Can you work these out from the model? Positions are in its coordinate system, mm. Face numbers are marked on the shaded views. A direction names the side the tool comes from. Round coordinates to 2 decimals unless told otherwise and drop trailing zeros.
Q1. For the marked faces 1 and 2, which set-ups out of +Z, -Z, +X, -X, +Y, -Y let a thin tool reach every point of the face, with its end or its side?
Q2. Will these pins go through, and if not, where does the flat tip stop? P1, Ø1.5, axis at y = 25, z = 1, coming from the -X side; P2, Ø3, axis at x = 15.5, z = 6, coming from the +Y side; P3, Ø2, axis at x = -1, z = 4.5, coming from the -Y side.
Q3. We'd pull the mould along X, two halves only. Please class the marked faces 3 and 4: pulls with the +X half, pulls with the -X half, needs draft (parallel to the pull), parting line crosses it, or undercut.
Q4. If we section it at A-A (x = 7.5): Count the separate pieces of the cut face and the enclosed holes in it, plus the area to 3 significant figures.
Q5. If I drill on line 1 (X direction, y = -0.5, z = 4.5); line 2 (Y direction, x = 7.5, z = 4); line 3 (Z direction, x = 22, y = 19.5), over which ranges is the centre line in solid material (lowest first)?
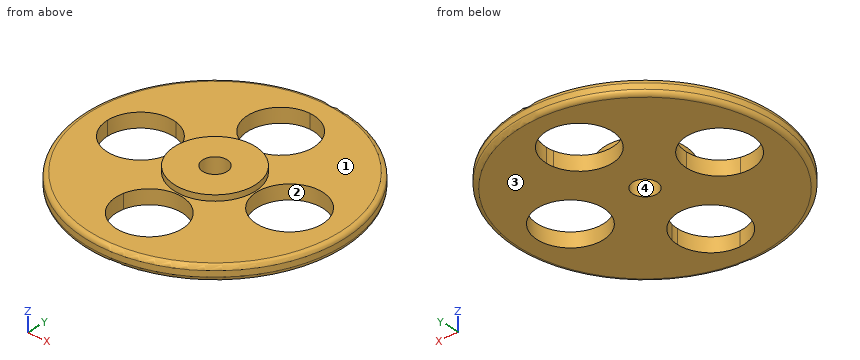
from build123d import *

# Parameters (mm, degrees)
F0_R     = 45
F0_R_2   = 14
F1_DEPTH = 5
F0_R_3   = 4.25
F2_DEPTH = 7
F3_R     = 1.5


with BuildPart() as f1:
    # F0 (on Top) → F1 (new body)
    with BuildSketch(Plane.XY):
        Circle(F0_R)
        with BuildLine():
            ThreePointArc((0, 37.5), (26.5165042945, 26.5165042945), (37.5, 0))
            ThreePointArc((37.5, 0), (26.5165043235, -26.5165042654), (8.22e-08, -37.5))
            ThreePointArc((8.22e-08, -37.5), (-26.516504245, -26.516504344), (-37.5, -5.77e-08))
            ThreePointArc((-37.5, -5.77e-08), (-26.5165043149, 26.5165042741), (0, 37.5))
        make_face(mode=Mode.SUBTRACT)
        with BuildLine():
            ThreePointArc((23.4567307692, -11.2152477289), (14.5, 0), (23.4567307692, 11.2152477289))
            ThreePointArc((23.4567307692, 11.2152477289), (18.3847763109, 18.3847763108), (11.2152477289, 23.4567307692))
            ThreePointArc((11.2152477289, 23.4567307692), (0, 14.5), (-11.2152477289, 23.4567307692))
            ThreePointArc((-11.2152477289, 23.4567307692), (-18.3847763109, 18.3847763108), (-23.4567307692, 11.2152477289))
            ThreePointArc((-23.4567307692, 11.2152477289), (-17.0139664992, 7.1764337887), (-14.5, 0))
            ThreePointArc((-14.5, 0), (-17.0139664992, -7.1764337887), (-23.4567307692, -11.2152477289))
            ThreePointArc((-23.4567307692, -11.2152477289), (-18.3847763109, -18.3847763108), (-11.2152477289, -23.4567307692))
            ThreePointArc((-11.2152477289, -23.4567307692), (0, -14.5), (11.2152477289, -23.4567307692))
            ThreePointArc((11.2152477289, -23.4567307692), (18.3847763109, -18.3847763108), (23.4567307692, -11.2152477289))
        make_face()
        Circle(F0_R_2, mode=Mode.SUBTRACT)
        with BuildLine():
            ThreePointArc((-11.2152477289, 23.4567307692), (-8.9860335008, 33.1764337887), (0, 37.5))
            ThreePointArc((0, 37.5), (-26.5165043149, 26.5165042741), (-37.5, -5.77e-08))
            ThreePointArc((-37.5, -5.77e-08), (-33.1764338112, 8.9860334828), (-23.4567307692, 11.2152477289))
            ThreePointArc((-23.4567307692, 11.2152477289), (-18.3847763109, 18.3847763108), (-11.2152477289, 23.4567307692))
        make_face()
        with BuildLine():
            ThreePointArc((23.4567307692, 11.2152477289), (33.1764337887, 8.9860335008), (37.5, 0))
            ThreePointArc((37.5, 0), (26.5165042945, 26.5165042945), (0, 37.5))
            ThreePointArc((0, 37.5), (8.1317279836, 34.1317279836), (11.5, 26))
            ThreePointArc((11.5, 26), (11.4285902211, 24.7204197723), (11.2152477289, 23.4567307692))
            ThreePointArc((11.2152477289, 23.4567307692), (18.3847763109, 18.3847763108), (23.4567307692, 11.2152477289))
        make_face()
        with BuildLine():
            ThreePointArc((-37.5, -5.77e-08), (-26.516504245, -26.516504344), (8.22e-08, -37.5))
            ThreePointArc((8.22e-08, -37.5), (-8.9860334751, -33.1764338208), (-11.2152477289, -23.4567307692))
            ThreePointArc((-11.2152477289, -23.4567307692), (-18.3847763109, -18.3847763108), (-23.4567307692, -11.2152477289))
            ThreePointArc((-23.4567307692, -11.2152477289), (-33.1764337661, -8.9860335188), (-37.5, -5.77e-08))
        make_face()
        with BuildLine():
            ThreePointArc((8.22e-08, -37.5), (26.5165043235, -26.5165042654), (37.5, 0))
            ThreePointArc((37.5, 0), (33.1764337887, -8.9860335008), (23.4567307692, -11.2152477289))
            ThreePointArc((23.4567307692, -11.2152477289), (18.3847763109, -18.3847763108), (11.2152477289, -23.4567307692))
            ThreePointArc((11.2152477289, -23.4567307692), (11.4285902211, -24.7204197723), (11.5, -26))
            ThreePointArc((11.5, -26), (8.1317280127, -34.1317279546), (8.22e-08, -37.5))
        make_face()
    extrude(amount=F1_DEPTH)

    # F0 (on Top) → F2 (join)
    with BuildSketch(Plane.XY):
        Circle(F0_R_2)
        Circle(F0_R_3, mode=Mode.SUBTRACT)
    extrude(amount=F2_DEPTH)

    # F3
    f3_edges = [f1.edges().sort_by_distance(p)[0] for p in [
        (-45, 0, 5),
        (-45, 0, 0),
    ]]
    fillet(f3_edges, radius=F3_R)


solid = f1.part
Solution:
1. face 1: +Z
1. face 2: +Z, -Z
2. P1: stops at x = -37.85
2. P2: stops at y = 41.93
2. P3: stops at y = -44.99
3. face 3: needs draft
3. face 4: undercut
4. separate pieces: 3
4. enclosed holes: 0
4. area: 315 mm2
5. line 1: x = -44.62 to -37.49, -14.51 to -4.22, 4.22 to 14.51, 37.49 to 44.62
5. line 2: y = -44.28 to -34.72, -17.28 to 17.28, 34.72 to 44.28
5. line 3: z = 0 to 5
